from build123d import *

# Parameters (mm, degrees)
EXTRUDE_1_DEPTH      = 4.360333
EXTRUDE_1_DEPTH_BACK = 4.360333
EXTRUDE_2_DEPTH      = 2
SKETCH_3_R           = 4.25
CUT_EXTRUDE_1_DEPTH  = 2


with BuildPart() as part:
    # Sketch 1 → Extrude 1 (new, two sides: drawn at the far end of the back side and taken through both)
    with BuildSketch(Plane(origin=(0, 0, 0), x_dir=(0, 0, -1), z_dir=(1, 0, 0)).offset(-EXTRUDE_1_DEPTH_BACK)):
        with BuildLine():
            Line((-11, 0), (-11, -4))
            Line((-11, -4), (-9, -4))
            Line((-9, -4), (-9, 0))
            Line((-9, 0), (9, 0))
            Line((9, 0), (9, -4))
            Line((9, -4), (11, -4))
            Line((11, -4), (11, 0))
            ThreePointArc((11, 0), (10.414213562, 1.414213562), (9, 2))
            Line((9, 2), (-9, 2))
            ThreePointArc((-9, 2), (-10.414213562, 1.414213562), (-11, 0))
        make_face()
    extrude(amount=EXTRUDE_1_DEPTH + EXTRUDE_1_DEPTH_BACK)

    # Sketch 2 → Extrude 2 (add)
    with BuildSketch(Plane(origin=(0, 0, 0), x_dir=(1, 0, 0), z_dir=(0, 1, 0))):
        with BuildLine():
            Line((-4.460661386, -8.95), (4.460661386, -8.95))
            ThreePointArc((4.460661386, -8.95), (10, 0), (4.460661386, 8.95))
            Line((4.460661386, 8.95), (-4.460661386, 8.95))
            ThreePointArc((-4.460661386, 8.95), (-10, 0), (-4.460661386, -8.95))
        make_face()
    extrude(amount=EXTRUDE_2_DEPTH)

    # Sketch 3 → Cut-Extrude 1 (cut)
    with BuildSketch(Plane(origin=(0, 0, 0), x_dir=(1, 0, 0), z_dir=(0, 1, 0))):
        with Locations(Location((0, 0, 0), (0, 0, 270))):
            Circle(SKETCH_3_R)
    extrude(amount=CUT_EXTRUDE_1_DEPTH, mode=Mode.SUBTRACT)


solid = part.part
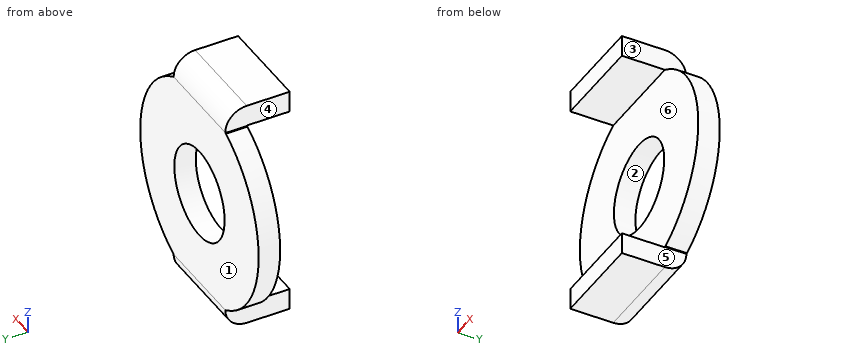
Work out the finished part from the listing and answer in its coordinate system (mm). Face numbers are marked on the shaded views. A direction names the side the tool comes from. Give positions to 0.01 mm unless a question says otherwise; leave off trailing zeros. Loops run counter-clockwise (first coordinate to the right, second up) from the corner with the lowest first, then second, coordinate; pieces in that order, holes last. Notation, with made-up numbers: (68.5, 68.25) - (79.5, 68.25) arc R13 cw to (79.5, 80.25) - close; hole circle Ø2 at (53.25, -36). An arc over 180 degrees is marked (long way). Answer in a Markdown table with one row per item.
(1) Consider L1, parallel to Z at x = -1, y = -2; L2, parallel to Y at x = 7, z = -3.5; L3, parallel to Z at x = -2.25, y = 0.4. Determine where each line is inside the solid, lowest interval first. Write a range as [from, to].
Results list:
| item | result |
|---|---|
| L1 | z = [-11, -9], [9, 11] |
| L2 | y = [0, 2] |
| L3 | z = [-10.96, -3.61], [3.61, 10.96] |
(2) Section D-D (x = -3) is taken. Give the vertices of the cut face in (y, z), and give its area (3 significant figures).
Results list:
| item | result |
|---|---|
| outline | (-4, -11) - (0, -11) arc R2 ccw to (2, -9) - (2, -3.01) - (0, -3.01) - (0, -9) - (-4, -9) - close; (-4, 9) - (0, 9) - (0, 3.01) - (2, 3.01) - (2, 9) arc R2 ccw to (0, 11) - (-4, 11) - close |
| area | 46.2 mm² |
(3) For a pull along X with two mould halves and no side action, classify the marked faces 1, 2 and 3 as pulls with the +X half, pulls with the -X half, needs draft (parallel to the pull), parting line crosses it, or undercut.
Results list:
| item | result |
|---|---|
| face 1 | needs draft |
| face 2 | undercut |
| face 3 | pulls with the +X half |
(4) Section C-C (x = 0) is taken. Give the vertices of the cut face in (y, z).
Results list:
| item | result |
|---|---|
| outline | (-4, -11) - (0, -11) arc R2 ccw to (2, -9) - (2, -4.25) - (0, -4.25) - (0, -9) - (-4, -9) - close; (-4, 9) - (0, 9) - (0, 4.25) - (2, 4.25) - (2, 9) arc R2 ccw to (0, 11) - (-4, 11) - close |
(5) A tool of negligible diameter and unlimited length cuts with its end or side. For the marked faces 4, 5 and 6, from which of +Z, -Z, +X, -X, +Y, -Y can it reach the whole face along a straight path? Write none if from no direction.
Results list:
| item | result |
|---|---|
| face 4 | +Z, -X, +Y, -Y |
| face 5 | -Z, +X, +Y, -Y |
| face 6 | +X, -X, -Y |
(6) Flat-ended cylindrical pins translate along their axes: pin 1 Ø9 at (x, z) = (-1.5, -3) entering from -Y; pin 2 Ø1 at (y, z) = (-2, -10.5) entering from -X; pin 3 Ø2.5 at (y, z) = (-1.5, -10.5) entering from +X; pin 4 Ø1.5 at (y, z) = (-2, 6) entering from +X. Find the tip coordinate at first contact, or state that the pin passes through.
Results list:
| item | result |
|---|---|
| pin 1 | stops at y = 0 |
| pin 2 | stops at x = -4.36 |
| pin 3 | stops at x = 4.36 |
| pin 4 | passes through |
(7) Section A-A (z = 0) is taken. Give the vertices of the cut face in (x, y), and give its area (3 significant figures).
Results list:
| item | result |
|---|---|
| outline | (-10, 0) - (-4.25, 0) - (-4.25, 2) - (-10, 2) - close; (4.25, 0) - (10, 0) - (10, 2) - (4.25, 2) - close |
| area | 23.0 mm² |
(8) Section B-B (y = -2.2) is taken. Give the vertices of the cut face in (x, z).
Results list:
| item | result |
|---|---|
| outline | (-4.36, -11) - (4.36, -11) - (4.36, -9) - (-4.36, -9) - close; (-4.36, 9) - (4.36, 9) - (4.36, 11) - (-4.36, 11) - close |
